For this review, take the finished solid that the model builds, in its own axes (mm). Face numbers are marked on the shaded views. A direction names the side the tool comes from. Round coordinates to 2 decimals unless told otherwise and drop trailing zeros. Write each loop counter-clockwise with the first axis right and the second up, starting at its lowest first coordinate (ties: lowest second). Pieces come first, ordered by that corner, then holes. Notation, with made-up numbers: M 46,15 L 84,15 A12 cw 84,37 Z; hole C 3.25,66.5 d8. An arc over 180 degrees is marked long. One line per question, with ' | ' between items.
Autodesk Inventor part; units mm, degrees
ref_plane "YZ Plane" through (0, 0, 0) normal (1, 0, 0) x (0, 1, 0)
ref_plane "XZ Plane" through (0, 0, 0) normal (0, 1, 0) x (-1, 0, 0)
ref_plane "XY Plane" through (0, 0, 0) normal (0, 0, 1) x (1, 0, 0)
sketch "Sketch1" plane through (0, 0, 0) normal (0, 0, 1) x (1, 0, 0)
  line L0 (-8.6606, 15.5596) -> (7.3394, 15.5596)
  line L1 (7.3394, 15.5596) -> (7.3394, -64.4404)
  line L2 (7.3394, -64.4404) -> (-8.6606, -64.4404)
  line L3 (-8.6606, -64.4404) -> (-8.6606, 15.5596)
  point P0 (0, 0)
  dimension "d2" = 16
  dimension "d3" = 80
extrude "Extrusion1" add sketch "Sketch1" along normal blind 16
sketch "Sketch2" plane through (-8.6606, 15.5596, 0) normal (0, 1, 0) x (1, 0, 0)
  line L0 (16, 0) -> (16, -16)
  line L1 (16, -11) -> (11, -11)
  line L2 (11, -11) -> (11, -5)
  line L3 (11, -5) -> (16, -5)
  line L4 (16, -5) -> (16, -11)
  line L5 (16, 0) -> (0, 0)
  line L6 (5, 0) -> (11, 0)
  line L7 (11, 0) -> (11, -5)
  line L8 (11, -5) -> (5, -5)
  line L9 (5, -5) -> (5, 0)
  line L10 (16, -16) -> (0, -16)
  line L11 (0, 0) -> (0, -16)
  point P0 (8.6606, 0)
  point P1 (5, -16)
  point P2 (0, -11)
  dimension "d5" = 5
  dimension "d6" = 5
  dimension "d7" = 5
  dimension "d8" = 5
  dimension "d9" = 5
  dimension "d10" = 5
extrude "Extrusion2" cut sketch "Sketch2" against normal blind 80 contours L0 L3 L7 L5 | L0 L1 L2 L3 | L7 L8 L9 L5
sketch "Sketch4" plane through (-8.6606, 15.5596, 16) normal (0, 1, 0) x (1, 0, 0)
  line L0 (6.9788, 8.1833) -> (8.6242, 5.3333)
  line L1 (8.6242, 5.3333) -> (6.9788, 2.4833)
  line L2 (6.9788, 2.4833) -> (3.6879, 2.4833)
  line L3 (3.6879, 2.4833) -> (2.0424, 5.3333)
  line L4 (2.0424, 5.3333) -> (3.6879, 8.1833)
  line L5 (3.6879, 8.1833) -> (6.9788, 8.1833)
  line L6 (16, 0) -> (0, 0)
  line L7 (0, 16) -> (0, 0)
  circle A0 centre (5.3333, 5.3333) radius 2.085
  point P0 (8.6606, 16)
  dimension "d13" = 5.3333
  dimension "d14" = 5.3333
  dimension "d15" = 5.7
  dimension "d23" = 4.17
extrude "Extrusion3" cut sketch "Sketch4" against normal blind 6 from surface at 0 contours A0
sketch "Sketch5" plane through (-8.6606, -64.4404, 16) normal (0, -1, 0) x (1, 0, 0)
  line L0 (3.6879, -2.4833) -> (2.0424, -5.3333)
  line L1 (3.6879, -2.4833) -> (6.9788, -2.4833)
  line L2 (6.9788, -2.4833) -> (8.6242, -5.3333)
  line L3 (8.6242, -5.3333) -> (6.9788, -8.1833)
  line L4 (6.9788, -8.1833) -> (3.6879, -8.1833)
  line L5 (3.6879, -8.1833) -> (2.0424, -5.3333)
  line L6 (2.0424, -5.3333) -> (3.6879, -2.4833)
  line L7 (0, 0) -> (16, 0)
  line L8 (0, -16) -> (0, 0)
  circle A0 centre (5.3333, -5.3333) radius 2.085
  point P0 (8.6606, -16)
  dimension "d18" = 5.3333
  dimension "d19" = 5.3333
  dimension "d24" = 4.17
extrude "Extrusion4" cut sketch "Sketch5" against normal blind 6 contours A0
fillet "Fillet2" radius 5 1 edges at (-8.6606, -24.4404, 16)
sketch "Sketch6" plane through (-3.6606, 15.5596, 5) normal (1, 0, 0) x (0, 0, -1)
  circle A0 centre (2.5, -10) radius 1.405
  line L0 (5, 0) -> (5, -80)
  line L1 (0, 0) -> (5, 0)
  point P0 (5, -15.5596)
  dimension "d25" = 2.81
  dimension "d26" = 2.5
  dimension "d27" = 10
extrude "Extrusion5" cut sketch "Sketch6" against normal blind 3
pattern_linear "Rectangular Pattern1" count 3 spacing 30 along (0, -1, 0) of "Extrusion5"
sketch "Sketch7" plane through (7.3394, 15.5596, 11) normal (0, 0, -1) x (-1, 0, 0)
  circle A0 centre (2.5, -10) radius 1.647
  line L0 (0, 0) -> (5, 0)
  line L1 (0, -80) -> (0, 0)
  point P0 (7.3394, -15.5596)
  dimension "d33" = 10
  dimension "d34" = 2.5
extrude "Extrusion6" cut sketch "Sketch7" against normal blind 3
pattern_linear "Rectangular Pattern2" count 3 spacing 30 along (0, -1, 0) of "Extrusion6"
equation "\"d2\" = SheetThickness + 2 * CornerOffset"
equation "\"d3\" = BoxHeight"
equation "\"d0\" = SheetThickness + 2 * CornerOffset"
equation "\"d5\" = CornerOffset"
equation "\"d6\" = CornerOffset"
equation "\"d7\" = CornerOffset"
equation "\"d8\" = CornerOffset"
equation "\"d9\" = CornerOffset"
equation "\"d10\" = CornerOffset"
equation "\"d11\" = BoxHeight"
equation "\"d15\" = NutS"
equation "\"d23\" = NutThreadD2"
equation "\"d16\" = NutThreadL"
equation "\"d24\" = NutThreadD2"
equation "\"d20\" = NutThreadL"
equation "\"d25\" = SideNutThreadd2"
equation "\"d26\" = SideNutWidth"
equation "\"d27\" = SideNutDistance"
equation "\"d33\" = SideNutDistance"
equation "\"d34\" = SideNutWidth"
equation "\"BoxHeight\" = 80"
equation "\"SheetThickness\" = 6"
equation "\"CornerOffset\" = 5"
equation "\"NutM\" = 2.7"
equation "\"NutS\" = 5.7"
equation "\"NutThreadD2\" = 4.17"
equation "\"NutThreadL\" = 6"
equation "\"SideNutThreadd2\" = 2.81"
equation "\"SideNutDistance\" = 10"
equation "\"SideNutWidth\" = 2.5"
properties part number "Corner"
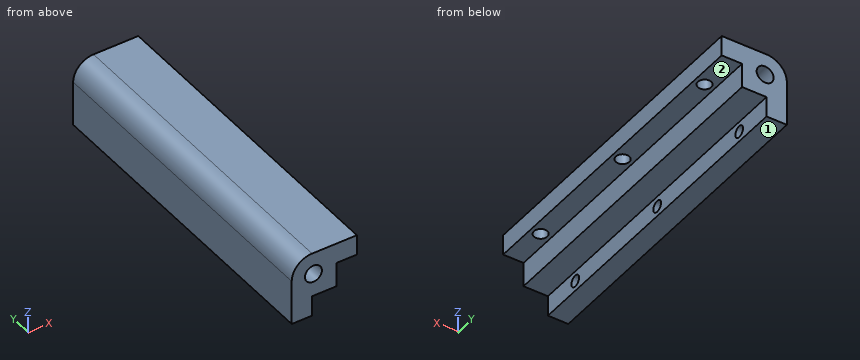
Item 1: Take a section at A-A (y = -21.5). Write out the cut boundary in (x, z), then the cut area to 3 significant figures.
Results:
outline: M -8.66,0 L -3.66,0 L -3.66,5 L 2.34,5 L 2.34,11 L 7.34,11 L 7.34,16 L -3.66,16 A5 ccw -8.66,11 Z | area: 166 mm2
Item 2: To check wall thickness, follow line 1 along Y through (x, z) = (-5.65, 2.5); line 2 along X through (y, z) = (0.5, 4.75); line 3 along Z through (x, y) = (-1.75, -46). State the ranges of each line that lie inside material, in increasing order. Write a range as from..to.
Results:
line 1: -64.44..-55.85, -53.04..-25.85, -23.04..4.15, 6.96..15.56 | line 2: -8.66..-3.66 | line 3: 5..16
Item 3: Take a section at C-C (x = 4.5). Write out the cut boundary in (y, z), then the cut area to 3 significant figures.
Results:
outline: M -64.44,11 L -56.05,11 L -56.05,14 L -52.83,14 L -52.83,11 L -26.05,11 L -26.05,14 L -22.83,14 L -22.83,11 L 3.95,11 L 3.95,14 L 7.17,14 L 7.17,11 L 15.56,11 L 15.56,16 L -64.44,16 Z | area: 371 mm2
Item 4: Machinability: for the marked faces 1 and 2, which of the approach directions +Z, -Z, +X, -X, +Y, -Y give a long, thin tool a straight path to every point of the face, cutting with its end or side? Answer none if there is none.
Results:
face 1: -Z, +X, -X, +Y, -Y | face 2: -Z, +X, +Y, -Y
Item 5: Take a section at D-D (x = 1). Write out the cut boundary in (y, z).
Results:
outline: M -64.44,5 L 15.56,5 L 15.56,16 L -64.44,16 Z
Item 6: Insertion check: pin 1 Ø6 at (y, z) = (-16, 5.5) entering from +X; pin 2 Ø3 at (x, y) = (-1.5, -15) entering from -Z; pin 3 Ø4 at (x, z) = (-3.33, 10.67) entering from -Y. Each pin has a flat end and moves straight along its axis. Give the tip position at first contact, or say it passes through.
Results:
pin 1: x = 2.34 | pin 2: z = 5 | pin 3: y = -58.44
Item 7: Take a section at B-B (z = 2.5). Write out the cut boundary in (x, y).
Results:
outline: M -8.66,-64.44 L -3.66,-64.44 L -3.66,-55.85 L -6.66,-55.85 L -6.66,-53.04 L -3.66,-53.04 L -3.66,-25.85 L -6.66,-25.85 L -6.66,-23.04 L -3.66,-23.04 L -3.66,4.15 L -6.66,4.15 L -6.66,6.96 L -3.66,6.96 L -3.66,15.56 L -8.66,15.56 Z
